Geometry check sheet. Reference: the model listing, model coordinates, mm. Round coordinates to 2 decimals unless told otherwise and drop trailing zeros. Write each loop counter-clockwise with the first axis right and the second up, starting at its lowest first coordinate (ties: lowest second). Pieces come first, ordered by that corner, then holes. Notation, with made-up numbers: (-22, -24) -> (30, -24) arc R11 cw to (30, -18) -> close; hole circle Ø2 at (46.25, -5.5). An arc over 180 degrees is marked (long way). Use a Markdown table: item, result.
```python
from build123d import *

# Parameters (mm, degrees)
SKETCH1_R           = 15
SKETCH1_R_2         = 10.5
BOSS_EXTRUDE1_DEPTH = 10
SKETCH2_R           = 15
BOSS_EXTRUDE2_DEPTH = 5
SKETCH3_R           = 10
BOSS_EXTRUDE3_DEPTH = 20
CHAMFER2_SIZE       = 2
FILLET1_R           = 2


with BuildPart() as part:
    # Sketch1 → Boss-Extrude1 (new body)
    with BuildSketch(Plane(origin=(0, 0, 0), x_dir=(1, 0, 0), z_dir=(0, 1, 0))):
        with Locations(Location((0, 0, 0), (0, 0, 270))):
            Circle(SKETCH1_R)
        with Locations(Location((0, 0, 0), (0, 0, 270))):
            Circle(SKETCH1_R_2, mode=Mode.SUBTRACT)
    extrude(amount=BOSS_EXTRUDE1_DEPTH)

    # Sketch2 → Boss-Extrude2 (add)
    with BuildSketch(Plane(origin=(0, 10, 0), x_dir=(1, 0, 0), z_dir=(0, 1, 0))):
        with Locations(Location((0, 0, 0), (0, 0, 270))):
            Circle(SKETCH2_R)
    extrude(amount=BOSS_EXTRUDE2_DEPTH)

    # Sketch3 → Boss-Extrude3 (add)
    with BuildSketch(Plane(origin=(0, 15, 0), x_dir=(1, 0, 0), z_dir=(0, 1, 0))):
        with Locations(Location((0, 0, 0), (0, 0, 270))):
            Circle(SKETCH3_R)
    extrude(amount=BOSS_EXTRUDE3_DEPTH)

    # Chamfer2
    chamfer2_edges = [part.edges().sort_by_distance(p)[0] for p in [
        (0, 35, -10),
    ]]
    chamfer(chamfer2_edges, length=CHAMFER2_SIZE)

    # Fillet1
    fillet1_edges = [part.edges().sort_by_distance(p)[0] for p in [
        (0, 0, -15),
        (0, 15, -15),
    ]]
    fillet(fillet1_edges, radius=FILLET1_R)


solid = part.part
```
(1) Section check D-D on y = 31. Record the cut outline in (x, z), plus the area to 3 significant figures.
A:
| item | result |
|---|---|
| outline | circle Ø20 at (0, 0) |
| area | 314 mm2 |
(2) Release check for a two-part mould opening along Z. For faces 1 (the face through (-9.76, 23.87, -2.17)), 2 (the face through (3.2, 4.9, 10)), 3 (the face through (-8, 15, 7)), 4 (the face through (0, 10, 0)) record: +Z half, -Z half, draft (parallel to the pull), parting line (faces both ways), or undercut.
A:
| item | result |
|---|---|
| face 1 | parting line |
| face 2 | undercut |
| face 3 | draft |
| face 4 | undercut |
(3) Gauge pin test, flat ends, axial feed: pin 1 Ø6 at (x, z) = (-1, 4) entering from -Y; pin 2 Ø1.5 at (y, z) = (30, -5) entering from -X; pin 3 Ø3 at (x, z) = (4, -9) entering from +Y; pin 4 Ø10 at (x, z) = (8, 2) entering from -Y. Record the tip position at first contact, or that the pin passes through.
A:
| item | result |
|---|---|
| pin 1 | stops at y = 10 |
| pin 2 | stops at x = -9.05 |
| pin 3 | stops at y = 34.65 |
| pin 4 | stops at y = 0 |
(4) Section check B-B on y = 5. Record the cut outline in (x, z), plus the area to 3 significant figures.
A:
| item | result |
|---|---|
| outline | circle Ø30 at (0, 0); hole circle Ø21 at (0, 0) |
| area | 360 mm2 |
(5) Thickness scan on line 1 (X direction, y = 6.25, z = 0); line 2 (Y direction, x = -2, z = -11.5); line 3 (X direction, y = 19.5, z = -0.25). Record the ranges inside material, lowest first.
A:
| item | result |
|---|---|
| line 1 | x = -15 to -10.5, 10.5 to 15 |
| line 2 | y = 0 to 15 |
| line 3 | x = -10 to 10 |
(6) Section check C-C on x = 0. Record the cut outline in (y, z).
A:
| item | result |
|---|---|
| outline | (0, -13) arc R2 ccw to (2, -15) -> (13, -15) arc R2 ccw to (15, -13) -> (15, -10) -> (33, -10) -> (35, -8) -> (35, 8) -> (33, 10) -> (15, 10) -> (15, 13) arc R2 ccw to (13, 15) -> (2, 15) arc R2 ccw to (0, 13) -> (0, 10.5) -> (10, 10.5) -> (10, -10.5) -> (0, -10.5) -> close |
(7) Section check A-A on z = 0. Record the cut outline in (x, y), plus the area to 3 significant figures.
A:
| item | result |
|---|---|
| outline | (-15, 2) arc R2 ccw to (-13, 0) -> (-10.5, 0) -> (-10.5, 10) -> (10.5, 10) -> (10.5, 0) -> (13, 0) arc R2 ccw to (15, 2) -> (15, 13) arc R2 ccw to (13, 15) -> (10, 15) -> (10, 33) -> (8, 35) -> (-8, 35) -> (-10, 33) -> (-10, 15) -> (-13, 15) arc R2 ccw to (-15, 13) -> close |
| area | 633 mm2 |
